For this review, take the finished solid that the model builds, in its own axes (mm). A direction names the side the tool comes from. Coordinates: 2 decimals unless noted, no trailing zeros. Loops run counter-clockwise (first coordinate to the right, second up) from the corner with the lowest first, then second, coordinate; pieces in that order, holes last. Notation, with made-up numbers: M 54.5,-20.75 L 95.5,-20.75 A21 ccw 95.5,17.25 Z; hole C -3,-25 d5. An arc over 180 degrees is marked long. Answer as a JSON object with one key per item and string values. Group by question number.
Item 1: Mouldability with a two-part tool opening along Y and no side actions: class faces 5 (the face through (11, -11, 12.7)), 6 (the face through (-7.955, -6.1, 8.988)), 7 (the face through (48.454, 15.259, 6.261)) as +Y half, -Y half, draft (parallel to the pull), parting line (faces both ways), or undercut.
Item 2: Insertion check: pin 1 (20.5 mm diameter, centred on x = 0, y = 0, fed in from +Z); pin 2 (1.1 mm diameter, centred on y = -1, z = 0.5, fed in from +X); pin 3 (0.5 mm diameter, centred on y = -3.5, z = 0.5, fed in from -X); pin 4 (3 mm diameter, centred on x = -34.5, y = -40.5, fed in from -Z). Each pin has a flat end and moves straight along its axis. Give the tip position at first contact, or say it passes through.
Item 3: Wall thickness on L1, parallel to Y at x = 0, z = 9.7 (3 decimals); L2, parallel to Y at x = 0, z = 5.25; L3, parallel to Y at x = 34, z = 4.5: over which ranges is each line inside the solid? List them lowest first. Write a range as from..to.
Item 4: Add section A-A (y = 0). State the section outline as (x, z) points (3 decimals), then the cut area to 3 significant figures.
Item 5: Add section C-C (z = 9). State the section outline as (x, y) points (3 decimals), then the cut area to 3 significant figures.
Item 6: Add section D-D (y = 15). State the section outline as (x, z) points, then the cut area to 3 significant figures.
Item 7: Tool access review of faces 1 (the face through (42, 0, 1)), 2 (the face through (-9, 12, 0)), 3 (the face through (-10.1, -7.7, 3.1)), 4 (the face through (-2, 10, 11.7)): name each direction out of +Z, -Z, +X, -X, +Y, -Y from which nothing blocks a thin tool from reaching the whole face with its end or side.
Item 8: Add section B-B (x = 0). State the section outline as (y, z) points (3 decimals), then the cut area to 3 significant figures.
from build123d import *

# Parameters (mm, degrees)
SKETCH1_R           = 50.8
SKETCH1_R_2         = 13.2
SKETCH1_R_3         = 10.025
SKETCH1_R_4         = 12.7
BOSS_EXTRUDE1_DEPTH = 12.7
CUT_EXTRUDE1_START  = 12.7
SKETCH1_3_R         = 13.2
SKETCH1_3_R_2       = 12.7
SKETCH1_3_R_3       = 10.025
CUT_EXTRUDE1_DEPTH  = 1
SKETCH1_4_R         = 12.7
SKETCH1_4_R_2       = 10.025
CUT_EXTRUDE2_DEPTH  = 6.35
CUT_EXTRUDE3_DEPTH  = 1


with BuildPart() as part:
    # Sketch1 → Boss-Extrude1 (new body)
    with BuildSketch(Plane(origin=(0, 0, 0), x_dir=(0, 1, 0), z_dir=(0, 0, 1))):
        with Locations(Location((0, 0, 0), (0, 0, 270))):
            Circle(SKETCH1_R)
        Circle(SKETCH1_R_2, mode=Mode.SUBTRACT)
        Circle(SKETCH1_R_2)
        with Locations(Location((0, 0, 0), (0, 0, 270))):
            Circle(SKETCH1_R_3, mode=Mode.SUBTRACT)
        Circle(SKETCH1_R_4)
        with Locations(Location((0, 0, 0), (0, 0, 270))):
            Circle(SKETCH1_R_3, mode=Mode.SUBTRACT)
    extrude(amount=BOSS_EXTRUDE1_DEPTH)

    # Sketch1<3> → Cut-Extrude1 (cut)
    with BuildSketch(Plane(origin=(0, 0, 0), x_dir=(0, 1, 0), z_dir=(0, 0, 1)).offset(CUT_EXTRUDE1_START)):
        with Locations(Location((0, 0, 0), (0, 0, 270))):
            Circle(SKETCH1_3_R)
        Circle(SKETCH1_3_R_2, mode=Mode.SUBTRACT)
        Circle(SKETCH1_3_R_2)
        with Locations(Location((0, 0, 0), (0, 0, 270))):
            Circle(SKETCH1_3_R_3, mode=Mode.SUBTRACT)
    extrude(amount=-CUT_EXTRUDE1_DEPTH, mode=Mode.SUBTRACT)

    # Sketch1<4> → Cut-Extrude2 (cut)
    with BuildSketch(Plane(origin=(0, 0, 0), x_dir=(0, 1, 0), z_dir=(0, 0, 1))):
        with Locations(Location((0, 0, 0), (0, 0, 270))):
            Circle(SKETCH1_4_R)
        with Locations(Location((0, 0, 0), (0, 0, 270))):
            Circle(SKETCH1_4_R_2, mode=Mode.SUBTRACT)
    extrude(amount=CUT_EXTRUDE2_DEPTH, mode=Mode.SUBTRACT)

    # Sketch2 → Cut-Extrude3 (cut)
    with BuildSketch(Plane(origin=(0, 0, 0), x_dir=(1, 0, 0), z_dir=(0, 0, -1))):
        with BuildLine():
            Line((-38.1, -33.601041651), (-38.1, 0))
            Line((-38.1, 0), (-38.1, 33.601041651))
            ThreePointArc((-38.1, 33.601041651), (-42.129575647, 28.385539555), (-45.45, 22.692234355))
            Line((-45.45, 22.692234355), (-45.45, -22.692234355))
            ThreePointArc((-45.45, -22.692234355), (-42.129575647, -28.385539555), (-38.1, -33.601041651))
        make_face()
        with BuildLine():
            ThreePointArc((45.45, 22.692234355), (42.129575647, 28.385539555), (38.1, 33.601041651))
            Line((38.1, 33.601041651), (38.1, 0))
            Line((38.1, 0), (38.1, -33.601041651))
            ThreePointArc((38.1, -33.601041651), (42.129575647, -28.385539555), (45.45, -22.692234355))
            Line((45.45, -22.692234355), (45.45, 22.692234355))
        make_face()
    extrude(amount=-CUT_EXTRUDE3_DEPTH, mode=Mode.SUBTRACT)


solid = part.part
From the geometry:
{
 "1": {"face 5": "draft", "face 6": "undercut", "face 7": "parting line"},
 "2": {"pin 1": "stops at z = 11.7", "pin 2": "stops at x = 50.8", "pin 3": "stops at x = -50.7", "pin 4": "passes through"},
 "3": {"L1": "y = -50.8..-10.025, 10.025..50.8", "L2": "y = -50.8..-12.7, 12.7..50.8", "L3": "y = -37.74..37.74"},
 "4": {"outline": "M -50.8,0 L -45.45,0 L -45.45,1 L -38.1,1 L -38.1,0 L -12.7,0 L -12.7,6.35 L -10.025,6.35 L -10.025,11.7 L -13.2,11.7 L -13.2,12.7 L -50.8,12.7 Z; M 10.025,6.35 L 12.7,6.35 L 12.7,0 L 38.1,0 L 38.1,1 L 45.45,1 L 45.45,0 L 50.8,0 L 50.8,12.7 L 13.2,12.7 L 13.2,11.7 L 10.025,11.7 Z", "area": "981 mm²"},
 "5": {"outline": "C 0,0 d101.6; hole C 0,0 d20.05", "area": "7,790 mm²"},
 "6": {"outline": "M -48.53,0 L -45.45,0 L -45.45,1 L -38.1,1 L -38.1,0 L 38.1,0 L 38.1,1 L 45.45,1 L 45.45,0 L 48.53,0 L 48.53,12.7 L -48.53,12.7 Z", "area": "1,220 mm²"},
 "7": {"face 1": "-Z, +Y, -Y", "face 2": "-Z, +X, -X, +Y, -Y", "face 3": "-Z", "face 4": "+Z"},
 "8": {"outline": "M -50.8,0 L -12.7,0 L -12.7,6.35 L -10.025,6.35 L -10.025,11.7 L -13.2,11.7 L -13.2,12.7 L -50.8,12.7 Z; M 10.025,6.35 L 12.7,6.35 L 12.7,0 L 50.8,0 L 50.8,12.7 L 13.2,12.7 L 13.2,11.7 L 10.025,11.7 Z", "area": "995 mm²"}
}
